Model file for the job. Use its own axes, mm. Round coordinates to 2 decimals unless told otherwise and drop trailing zeros. Loops run counter-clockwise (first coordinate to the right, second up) from the corner with the lowest first, then second, coordinate; pieces in that order, holes last. Notation, with made-up numbers: (33, -16) - (68, -16) arc R22 cw to (68, 6) - close; hole circle Ø8 at (86.5, -0.75). An arc over 180 degrees is marked (long way). Use one line per item in the form item = value.
from build123d import *

# Parameters (mm, degrees)
BOSS_EXTRUDE1_DEPTH             = 5
M5X0_8_TAPPED_HOLE1_D           = 4.2
M5X0_8_TAPPED_HOLE1_DEPTH       = 40
M5X0_8_TAPPED_HOLE1_CSINK_D     = 5.05
M5X0_8_TAPPED_HOLE1_CSINK_ANGLE = 90
M5X0_8_TAPPED_HOLE1_TIP         = 1.2618073
M5X0_8_TAPPED_HOLE2_D           = 4.2
M5X0_8_TAPPED_HOLE2_DEPTH       = 20.875
M5X0_8_TAPPED_HOLE2_CSINK_D     = 5.05
M5X0_8_TAPPED_HOLE2_CSINK_ANGLE = 90
F_1_4_0_25_DIAMETER_HOLE1_D     = 6.35
FILLET1_R                       = 5


with BuildPart() as part:
    # Sketch1 → Boss-Extrude1 (new body, symmetric)
    with BuildSketch(Plane(origin=(0, 0, 0), x_dir=(1, 0, 0), z_dir=(0, 1, 0))):
        with BuildLine():
            Line((-120.190475132, 51.601117357), (-99.684378478, 31.095020703))
            Line((-99.684378478, 31.095020703), (-106.75544629, 24.023952891))
            Line((-106.75544629, 24.023952891), (-41.365746699, -41.365746699))
            ThreePointArc((-41.365746699, -41.365746699), (8.808484383, -57.833040754), (51.805109545, -27.175))
            Line((51.805109545, -27.175), (79.375, -27.175))
            Line((79.375, -27.175), (79.375, 27.175))
            Line((79.375, 27.175), (51.805109545, 27.175))
            ThreePointArc((51.805109545, 27.175), (30.269724974, 50.059901618), (0, 58.5))
            Line((0, 58.5), (-113.291592489, 58.5))
            Line((-113.291592489, 58.5), (-120.190475132, 51.601117357))
        make_face()
        with BuildLine():
            Line((58.5, -14.5), (58.5, 14.5))
            Line((58.5, 14.5), (46.281745862, 14.5))
            ThreePointArc((46.281745862, 14.5), (-48.5, 0), (46.281745862, -14.5))
            Line((46.281745862, -14.5), (58.5, -14.5))
        make_face(mode=Mode.SUBTRACT)
        with BuildLine():
            Line((-92.613310666, 24.023952891), (-57.4247459, -11.164611875))
            ThreePointArc((-57.4247459, -11.164611875), (-56.48621622, 15.217009469), (-44.045431091, 38.5))
            Line((-44.045431091, 38.5), (-78.137263557, 38.5))
            Line((-78.137263557, 38.5), (-92.613310666, 24.023952891))
        make_face(mode=Mode.SUBTRACT)
    extrude(amount=BOSS_EXTRUDE1_DEPTH, both=True)

    # M5x0.8 Tapped Hole1
    with Locations(Plane(origin=(-34.294678888, 0, 34.294678888), x_dir=(0.707106781, 0, 0.707106781), z_dir=(-0.707106781, 0, 0.707106781))):
        with Locations((-116.475, 0), (-97.475, 0)):
            CounterSinkHole(M5X0_8_TAPPED_HOLE1_D / 2, M5X0_8_TAPPED_HOLE1_CSINK_D / 2, depth=M5X0_8_TAPPED_HOLE1_DEPTH, counter_sink_angle=M5X0_8_TAPPED_HOLE1_CSINK_ANGLE)
            with Locations((0, 0, -(M5X0_8_TAPPED_HOLE1_DEPTH + M5X0_8_TAPPED_HOLE1_TIP / 2))):  # 118° drill point
                Cone(0, M5X0_8_TAPPED_HOLE1_D / 2, M5X0_8_TAPPED_HOLE1_TIP, mode=Mode.SUBTRACT)

    # M5x0.8 Tapped Hole2
    with Locations(Plane.ZY.offset(-58.5)):
        with Locations((-9.5, 0), (9.5, 0)):
            CounterSinkHole(M5X0_8_TAPPED_HOLE2_D / 2, M5X0_8_TAPPED_HOLE2_CSINK_D / 2, depth=M5X0_8_TAPPED_HOLE2_DEPTH, counter_sink_angle=M5X0_8_TAPPED_HOLE2_CSINK_ANGLE)

    # 1/4 (0.25) Diameter Hole1 (through all)
    with Locations(Plane(origin=(0, 5, 0), x_dir=(1, 0, 0), z_dir=(0, 1, 0))):
        with Locations((71.2, 19), (71.2, 0), (71.2, -19)):
            Hole(F_1_4_0_25_DIAMETER_HOLE1_D / 2)

    # Fillet1
    fillet1_edges = [part.edges().sort_by_distance(p)[0] for p in [
        (-113.291592489, 0, -58.5),
        (51.805109545, 0, -27.175),
        (79.375, 0, -27.175),
        (79.375, 0, 27.175),
        (51.805109545, 0, 27.175),
        (46.281745862, 0, 14.5),
        (46.281745862, 0, -14.5),
        (-92.613310666, 0, -24.023952891),
        (-78.137263557, 0, -38.5),
        (-44.045431091, 0, -38.5),
        (-57.4247459, 0, 11.164611875),
    ]]
    fillet(fillet1_edges, radius=FILLET1_R)


solid = part.part
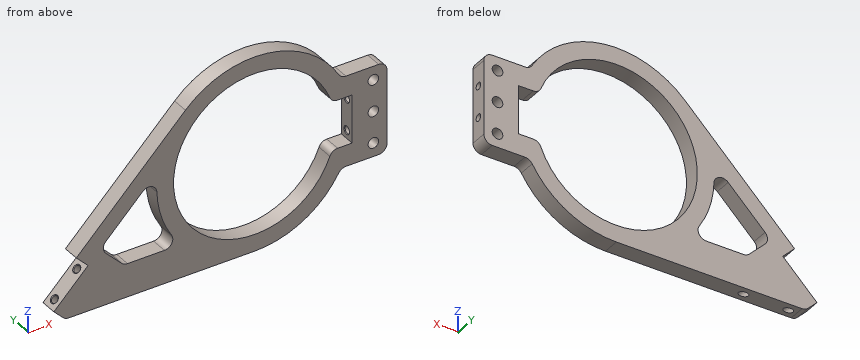
1. Cut at D-D, the plane y = 0. Give the number of separate pieces and of enclosed holes in the cut face, plus the area to 3 significant figures.
Geometry check:
separate_pieces = 4
enclosed_holes = 4
area = 6,470 mm^2
2. Cut at A-A, the plane z = 9.5. Give the cut face in (x, y) (1 decimal), plus the area to 3 significant figures.
Geometry check:
outline = (-73.2, -5) - (-47.6, -5) - (-47.6, 5) - (-73.2, 5) - close; (58.5, -5) - (79.4, -5) - (79.4, -2.1) - (58.9, -2.1) - (58.5, -2.5) - close; (58.5, 2.5) - (58.9, 2.1) - (79.4, 2.1) - (79.4, 5) - (58.5, 5) - close
area = 378 mm^2
3. Cut at C-C, the plane z = 38.5. Give the cut face in (x, y).
Geometry check:
outline = (-44.23, -5) - (-29.5, -5) - (-29.5, 5) - (-44.23, 5) - close; (29.5, -5) - (44.05, -5) - (44.05, 5) - (29.5, 5) - close
4. Wall check: probe 1 along Z at (x, y) = (71.2, 1) (3 decimals); probe 2 along X at (y, z) = (-1.5, 19) (1 decimal); probe 3 along Z at (x, y) = (71.2, -0.5) (3 decimals). Give the ranges that are in metal, low to high.
Geometry check:
probe_1 = -27.175 to -22.175, -15.825 to -11.347, -7.653 to -3.175, 3.175 to 7.653, 11.347 to 15.825, 22.175 to 27.175
probe_2 = -63.7 to -44.6, 44.6 to 68, 74.4 to 79.4
probe_3 = -27.175 to -22.175, -15.825 to -11.54, -7.46 to -3.175, 3.175 to 7.46, 11.54 to 15.825, 22.175 to 27.175
5. Flat gauge pins, fed straight in: pin 1 (6 mm diameter, centred on x = 32.5, y = -3, fed in from -Z); pin 2 (1 mm diameter, centred on x = 42, y = 2, fed in from -Z); pin 3 (5 mm diameter, centred on x = 42.5, y = -0.5, fed in from +Z); pin 4 (5 mm diameter, centred on x = 71.2, z = -19, fed in from -Y). Where does each tip first touch, or does it go through?
Geometry check:
pin_1 = -50.52
pin_2 = -41.23
pin_3 = 42.69
pin_4 = through
6. Cut at B-B, the plane x = 16. Give the cut face in (y, z), plus the area to 3 significant figures.
Geometry check:
outline = (-5, -56.27) - (5, -56.27) - (5, -45.78) - (-5, -45.78) - close; (-5, 45.78) - (5, 45.78) - (5, 56.27) - (-5, 56.27) - close
area = 210 mm^2
